The model under review builds one solid part; all positions refer to its coordinate system, in mm. Face numbers are marked on the shaded views. A direction names the side the tool comes from. Give positions to 0.01 mm unless a question says otherwise; leave off trailing zeros. Order: outer loops, then holes, each group sorted by start corner. A loop starts at its lowest first (then second) coordinate and runs counter-clockwise, first axis right, second up. Notation, with made-up numbers: (7.25, 66.25) - (36.25, 66.25) arc R24 ccw to (36.25, 104.25) - close; hole circle Ø8 at (58.25, 45.5). An arc over 180 degrees is marked (long way). Use a Markdown table: item, result. Add a question column.
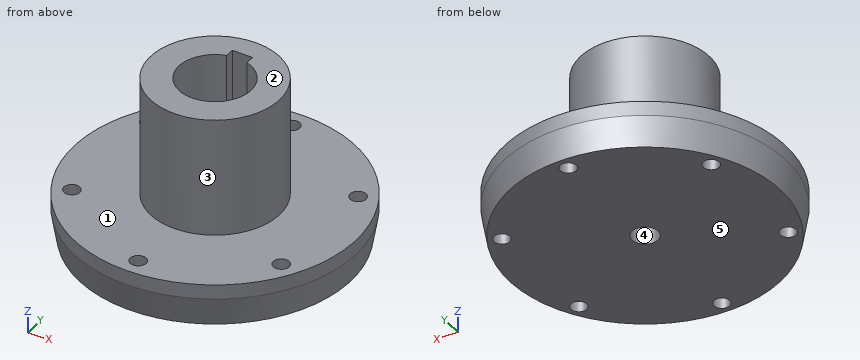
```python
from build123d import *

# Parameters (mm, degrees)
ESQUISSE1_R             = 54.5
BOSS_EXTRU_1_DEPTH      = 17
ESQUISSE5_R             = 25
BOSS_EXTRU_4_DEPTH      = 46
ENL_V_MAT_EXTRU_2_DEPTH = 56
ESQUISSE8_R             = 5.1
ENL_V_MAT_EXTRU_3_DEPTH = 76
ESQUISSE9_R             = 3.1
ENL_V_MAT_EXTRU_4_DEPTH = 76
CHANFREIN1_SIZE         = 2
CHANFREIN1_SIZE2        = 11.342563639


with BuildPart() as part:
    # Esquisse1 → Boss.-Extru.1 (new body)
    with BuildSketch(Plane.XY):
        Circle(ESQUISSE1_R)
    extrude(amount=BOSS_EXTRU_1_DEPTH)

    # Esquisse5 → Boss.-Extru.4 (add)
    with BuildSketch(Plane.XY.offset(17)):
        Circle(ESQUISSE5_R)
    extrude(amount=BOSS_EXTRU_4_DEPTH)

    # Esquisse7 → Enlèv. mat.-Extru.2 (cut)
    with BuildSketch(Plane.XY.offset(63)):
        with BuildLine():
            Line((-4, 17), (-4, 13.416407865))
            ThreePointArc((-4, 13.416407865), (0, -14), (4, 13.416407865))
            Line((4, 13.416407865), (4, 17))
            Line((4, 17), (-4, 17))
        make_face()
    extrude(amount=-ENL_V_MAT_EXTRU_2_DEPTH, mode=Mode.SUBTRACT)

    # Esquisse8 → Enlèv. mat.-Extru.3 (cut)
    with BuildSketch(Plane(origin=(0, 0, 0), x_dir=(-1, 0, 0), z_dir=(0, 0, -1))):
        Circle(ESQUISSE8_R)
    extrude(amount=-ENL_V_MAT_EXTRU_3_DEPTH, mode=Mode.SUBTRACT)

    # Esquisse9 → Enlèv. mat.-Extru.4 (cut)
    with BuildSketch(Plane(origin=(0, 0, 0), x_dir=(-1, 0, 0), z_dir=(0, 0, -1))):
        with Locations((0, 47.5)):
            Circle(ESQUISSE9_R)
        with Locations((41.13620668, 23.75)):
            Circle(ESQUISSE9_R)
        with Locations((41.13620668, -23.75)):
            Circle(ESQUISSE9_R)
        with Locations((0, -47.5)):
            Circle(ESQUISSE9_R)
        with Locations((-41.13620668, -23.75)):
            Circle(ESQUISSE9_R)
        with Locations((-41.13620668, 23.75)):
            Circle(ESQUISSE9_R)
    extrude(amount=-ENL_V_MAT_EXTRU_4_DEPTH, mode=Mode.SUBTRACT)

    # Chanfrein1
    chanfrein1_edges = [part.edges().sort_by_distance(p)[0] for p in [
        (-54.5, 0, 0),
    ]]
    chanfrein1_side = [part.faces().sort_by_distance(p)[0] for p in [
        (-52.958507217, 0, 0),
    ]]
    chamfer(chanfrein1_edges, length=CHANFREIN1_SIZE, length2=CHANFREIN1_SIZE2, reference=chanfrein1_side[0])


solid = part.part
```
Q1. We need section B-B (x = 0). Write out the cut boundary in (y, z).
Q2. We need section D-D (z = 9.5). Write out the cut boundary in (x, y).
Q3. We need section A-A (y = 0). Write out the cut boundary in (x, z), plus the area to 3 significant figures.
Q4. Draft analysis for pull direction Y (two halves, no side actions). For the marked faces 3, 4 and 5, state which applies: pulls with the +Y half, pulls with the -Y half, needs draft (parallel to the pull), parting line crosses it, or undercut.
Q5. Machinability: for the marked faces 1 and 2, which of the approach directions +Z, -Z, +X, -X, +Y, -Y give a long, thin tool a straight path to every point of the face, cutting with its end or side? Answer none if there is none.
Q6. Wall thickness on probe 1 along Y at (x, z) = (0, 27); probe 2 along Y at (x, z) = (0, 2); probe 3 along Y at (x, z) = (0, 3.25): over which ranges is each line inside the solid? List them lowest first.
Q7. Clearance check with flat-ended pins moving along their axes: P1, Ø12, axis at x = 26, z = 26, coming from the -Y side; P2, Ø11.5, axis at x = 0, y = 0, coming from the +Z side; P3, Ø5.5, axis at x = -41.14, y = 23.75, coming from the +Z side; P4, Ø1.1, axis at y = 15.5, z = 35, coming from the -X side. State where each tip first meets the part, or that it passes through.
Q8. We need section C-C (z = 45.5). Write out the cut boundary in (x, y).
Here are the results:
| question | item | result |
|---|---|---|
| 1 | outline | (-54.5, 11.34) - (-52.5, 0) - (-50.6, 0) - (-50.6, 17) - (-54.5, 17) - close; (-44.4, 0) - (-5.1, 0) - (-5.1, 7) - (-14, 7) - (-14, 63) - (-25, 63) - (-25, 17) - (-44.4, 17) - close; (5.1, 0) - (44.4, 0) - (44.4, 17) - (25, 17) - (25, 63) - (17, 63) - (17, 7) - (5.1, 7) - close; (50.6, 0) - (52.5, 0) - (54.5, 11.34) - (54.5, 17) - (50.6, 17) - close |
| 2 | outline | circle Ø108.35 at (0, 0); hole circle Ø6.2 at (-41.14, -23.75); hole circle Ø6.2 at (-41.14, 23.75); hole (-4, 13.42) arc R14 ccw (long way) to (4, 13.42) - (4, 17) - (-4, 17) - close; hole circle Ø6.2 at (0, -47.5); hole circle Ø6.2 at (0, 47.5); hole circle Ø6.2 at (41.14, -23.75); hole circle Ø6.2 at (41.14, 23.75) |
| 3 | outline | (-54.5, 11.34) - (-52.5, 0) - (-5.1, 0) - (-5.1, 7) - (-14, 7) - (-14, 63) - (-25, 63) - (-25, 17) - (-54.5, 17) - close; (5.1, 0) - (52.5, 0) - (54.5, 11.34) - (54.5, 17) - (25, 17) - (25, 63) - (14, 63) - (14, 7) - (5.1, 7) - close |
| 3 | area | 2,490 mm2 |
| 4 | face 3 | parting line crosses it |
| 4 | face 4 | undercut |
| 4 | face 5 | needs draft |
| 5 | face 1 | +Z |
| 5 | face 2 | +Z, +X, -X, +Y, -Y |
| 6 | probe 1 | -25 to -14, 17 to 25 |
| 6 | probe 2 | -52.85 to -50.6, -44.4 to -5.1, 5.1 to 44.4, 50.6 to 52.85 |
| 6 | probe 3 | -53.07 to -50.6, -44.4 to -5.1, 5.1 to 44.4, 50.6 to 53.07 |
| 7 | P1 | y = -15 |
| 7 | P2 | z = 7 |
| 7 | P3 | through |
| 7 | P4 | x = -20.04 |
| 8 | outline | circle Ø50 at (0, 0); hole (-4, 13.42) arc R14 ccw (long way) to (4, 13.42) - (4, 17) - (-4, 17) - close |
